from build123d import *

# Parameters (mm, degrees)
F0_W     = 2057.4
F0_H     = 914.4
F1_DEPTH = 914.4
F2_W     = 1752.6
F2_H     = 685.8
F3_DEPTH = 457.2
F4_R     = 30.48


with BuildPart() as f1:
    # F0 (on Top) → F1 (new body)
    with BuildSketch(Plane.XY):
        Rectangle(F0_W, F0_H)
    extrude(amount=F1_DEPTH)

    # F2 (on face) → F3 (cut)
    with BuildSketch(Plane.XY.offset(914.4)):
        with Locations((0, -114.3)):
            Rectangle(F2_W, F2_H)
    extrude(amount=-F3_DEPTH, mode=Mode.SUBTRACT)

    # F4
    f4_edges = [f1.edges().sort_by_distance(p)[0] for p in [
        (876.3, -114.3, 457.2),
        (0, 228.6, 457.2),
        (-876.3, -114.3, 457.2),
        (0, -457.2, 457.2),
        (-876.3, 228.6, 685.8),
        (-876.3, -457.2, 685.8),
        (-876.3, -114.3, 914.4),
        (876.3, 228.6, 685.8),
        (0, 228.6, 914.4),
        (0, -457.2, 0),
        (1028.7, -457.2, 457.2),
        (952.5, -457.2, 914.4),
        (876.3, -457.2, 685.8),
        (-952.5, -457.2, 914.4),
        (-1028.7, -457.2, 457.2),
        (-1028.7, 0, 914.4),
        (0, 457.2, 914.4),
        (1028.7, 0, 914.4),
        (876.3, -114.3, 914.4),
        (1028.7, 457.2, 457.2),
        (1028.7, 0, 0),
        (-1028.7, 457.2, 457.2),
        (-1028.7, 0, 0),
        (0, 457.2, 0),
    ]]
    fillet(f4_edges, radius=F4_R)


solid = f1.part
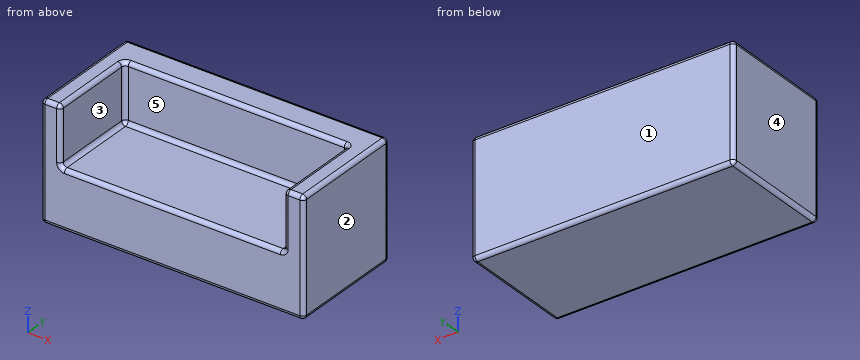
Design review of the part built by this model. Coordinates are the model's own, in mm. Face numbers are marked on the shaded views. A direction names the side the tool comes from. Give positions to 0.01 mm unless a question says otherwise; leave off trailing zeros. Order: outer loops, then holes, each group sorted by start corner. A loop starts at its lowest first (then second) coordinate and runs counter-clockwise, first axis right, second up.
1. Mouldability with a two-part tool opening along X and no side actions: class the marked faces 1, 2 and 3 as +X half, -X half, draft (parallel to the pull), parting line (faces both ways), or undercut.
Solution:
face 1: draft
face 2: +X half
face 3: undercut
2. To check wall thickness, follow L1, parallel to X at y = 28, z = 781.5; L2, parallel to Y at x = -265.5, z = 683; L3, parallel to Z at x = 635.5, y = 110.5. State the ranges of each line that lie inside material, in increasing order.
Solution:
L1: x = -1028.7 to -876.3, 876.3 to 1028.7
L2: y = 228.6 to 457.2
L3: z = 0 to 457.2
3. Add section A-A, the plane y = -198.5. State the section outline as (x, z) points.
Solution:
outline: (-1028.7, 30.48) arc R30.48 ccw to (-998.22, 0) - (998.22, 0) arc R30.48 ccw to (1028.7, 30.48) - (1028.7, 883.92) arc R30.48 ccw to (998.22, 914.4) - (906.78, 914.4) arc R30.48 ccw to (876.3, 883.92) - (876.3, 487.68) arc R30.48 cw to (845.82, 457.2) - (-845.82, 457.2) arc R30.48 cw to (-876.3, 487.68) - (-876.3, 883.92) arc R30.48 ccw to (-906.78, 914.4) - (-998.22, 914.4) arc R30.48 ccw to (-1028.7, 883.92) - close
4. Add section C-C, the plane x = 272.5. State the section outline as (y, z) points, then the cut area to 3 significant figures.
Solution:
outline: (-457.2, 30.48) arc R30.48 ccw to (-426.72, 0) - (426.72, 0) arc R30.48 ccw to (457.2, 30.48) - (457.2, 883.92) arc R30.48 ccw to (426.72, 914.4) - (259.08, 914.4) arc R30.48 ccw to (228.6, 883.92) - (228.6, 487.68) arc R30.48 cw to (198.12, 457.2) - (-426.72, 457.2) arc R30.48 ccw to (-457.2, 426.72) - close
area: 522,000 mm2
5. Add section B-B, the plane z = 725. State the section outline as (x, y) points, then the cut area to 3 significant figures.
Solution:
outline: (-1028.7, -426.72) arc R30.48 ccw to (-998.22, -457.2) - (-906.78, -457.2) arc R30.48 ccw to (-876.3, -426.72) - (-876.3, 198.12) arc R30.48 cw to (-845.82, 228.6) - (845.82, 228.6) arc R30.48 cw to (876.3, 198.12) - (876.3, -426.72) arc R30.48 ccw to (906.78, -457.2) - (998.22, -457.2) arc R30.48 ccw to (1028.7, -426.72) - (1028.7, 426.72) arc R30.48 ccw to (998.22, 457.2) - (-998.22, 457.2) arc R30.48 ccw to (-1028.7, 426.72) - close
area: 679,000 mm2
6. Tool access review of the marked faces 4 and 5: name each direction out of +Z, -Z, +X, -X, +Y, -Y from which nothing blocks a thin tool from reaching the whole face with its end or side.
Solution:
face 4: +Z, -Z, -X, +Y, -Y
face 5: +Z, -Y
7. For pin 1 Ø1.5 at (x, z) = (271.5, 760) entering from -Y; pin 2 Ø6 at (x, y) = (818.5, -175) entering from +Z, all flat-tipped, find the tip position at first contact; note any pin that passes through.
Solution:
pin 1: stops at y = 228.6
pin 2: stops at z = 457.2
